Input: dimensioned drawing with shaded views. Units: mm. Origin: part minimum x, y, z. Coordinates: 2 decimals unless noted, no trailing zeros. Order: outer loops, then holes, each group sorted by start corner. A loop starts at its lowest first (then second) coordinate and runs counter-clockwise, first axis right, second up. Notation, with made-up numbers: (19.25, 72.25) -> (65.25, 72.25) arc R35 ccw to (65.25, 109.25) -> close; hole circle Ø2 at (5.25, 72.25). An arc over 180 degrees is marked (long way). Write item = value, one per line. Start each with the question number.
Item 1: Contact query for flat-ended pins moving along their axis: pin 1 (8 mm diameter, centred on x = 16.42, y = 16.42, fed in from -Z); pin 2 (1.6 mm diameter, centred on y = 35.5, z = 1, fed in from +X); pin 3 (1 mm diameter, centred on x = 48, z = 1.5, fed in from +Y). Output: stop coordinate, or through.
Item 2: Ray query, line 1 along X through (y, z) = (33, 1.95); line 2 along X through (y, z) = (13, 0.9). Return the intervals inside material, ascending. Write a range as [from, to].
Item 3: Section query A-A (y = 44.45). Output: boundary loops of the cut face in (x, z) (1 decimal).
Item 4: Mould query, pull axis X, two halves, no side actions, for the marked faces 1 and 2. Classes: released by +X, released by -X, zero draft, split by the parting line, or undercut.
Item 5: Section query B-B (x = 12.7). Count the separate pieces of the cut face and the enclosed holes in it, then the cut area to 3 significant figures.
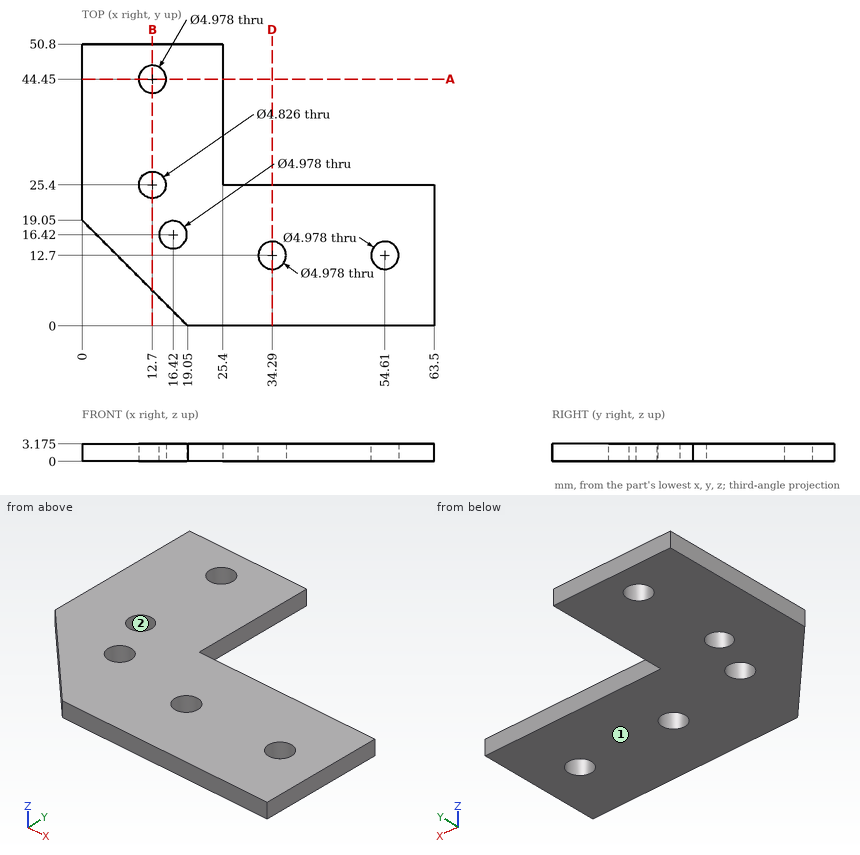
Computed:
q1.pin_1 = 0
q1.pin_2 = 25.4
q1.pin_3 = 25.4
q2.line_1 = [0, 25.4]
q2.line_2 = [6.05, 31.82], [36.76, 52.14], [57.08, 63.5]
q3.outline = (0, 0) -> (10.2, 0) -> (10.2, 3.2) -> (0, 3.2) -> close; (15.2, 0) -> (25.4, 0) -> (25.4, 3.2) -> (15.2, 3.2) -> close
q4.face_1 = zero draft
q4.face_2 = undercut
q5.separate_pieces = 3
q5.enclosed_holes = 0
q5.area = 110 mm^2
